from build123d import *

# Parameters (mm, degrees)
SKETCH1_W           = 275
SKETCH1_H           = 200
BOSS_EXTRUDE1_DEPTH = 1.5
SKETCH3_W           = 275
SKETCH3_H           = 200
SKETCH3_W_2         = 272
SKETCH3_H_2         = 197
BOSS_EXTRUDE2_DEPTH = 55
SKETCH4_R           = 1.5
SKETCH4_R_2         = 6.1
MOUNT_HOLE_DEPTH    = 250


with BuildPart() as part:
    # Sketch1 → Boss-Extrude1 (new body)
    with BuildSketch(Plane(origin=(0, 0, 0), x_dir=(1, 0, 0), z_dir=(0, 1, 0))):
        Rectangle(SKETCH1_W, SKETCH1_H)
    extrude(amount=BOSS_EXTRUDE1_DEPTH)

    # Sketch3 → Boss-Extrude2 (add)
    with BuildSketch(Plane(origin=(0, 1.5, 0), x_dir=(1, 0, 0), z_dir=(0, 1, 0))):
        Rectangle(SKETCH3_W, SKETCH3_H)
        Rectangle(SKETCH3_W_2, SKETCH3_H_2, mode=Mode.SUBTRACT)
    extrude(amount=BOSS_EXTRUDE2_DEPTH)

    # Sketch4 → MOUNT HOLE (cut)
    with BuildSketch(Plane(origin=(0, 0, -100), x_dir=(-1, 0, 0), z_dir=(0, 0, -1))):
        with Locations((-47, 28.25)):
            Circle(SKETCH4_R)
        with Locations((-54.75, 14.826606241)):
            Circle(SKETCH4_R)
        with Locations((-70.25, 14.826606241)):
            Circle(SKETCH4_R)
        with Locations((-78, 28.25)):
            Circle(SKETCH4_R)
        with Locations((-70.25, 41.673393759)):
            Circle(SKETCH4_R)
        with Locations((-54.75, 41.673393759)):
            Circle(SKETCH4_R)
        with Locations((78, 28.25)):
            Circle(SKETCH4_R)
        with Locations((70.25, 14.826606241)):
            Circle(SKETCH4_R)
        with Locations((54.75, 14.826606241)):
            Circle(SKETCH4_R)
        with Locations((47, 28.25)):
            Circle(SKETCH4_R)
        with Locations((54.75, 41.673393759)):
            Circle(SKETCH4_R)
        with Locations((70.25, 41.673393759)):
            Circle(SKETCH4_R)
        with Locations((-62.5, 21.5)):
            Circle(SKETCH4_R_2)
        with Locations((62.5, 21.5)):
            Circle(SKETCH4_R_2)
    extrude(amount=-MOUNT_HOLE_DEPTH, mode=Mode.SUBTRACT)


solid = part.part
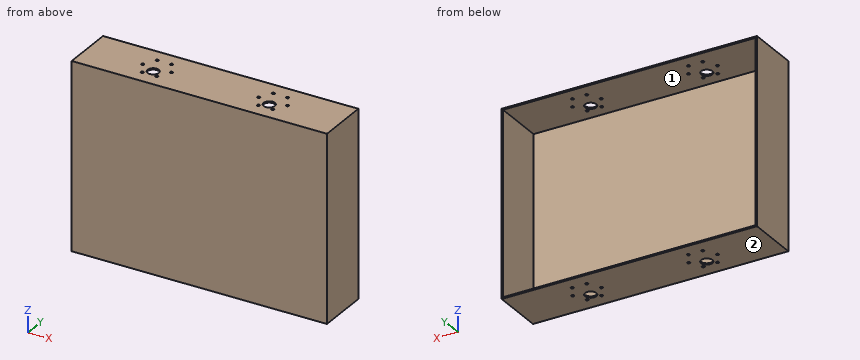
Read the model definition and answer for the solid it produces. Units are mm, in the model's axes. Face numbers are marked on the shaded views. A direction names the side the tool comes from. Give positions to 0.01 mm unless a question says otherwise; leave off trailing zeros. Write each loop counter-clockwise with the first axis right and the second up, starting at its lowest first coordinate (ties: lowest second). Pieces come first, ordered by that corner, then holes. Notation, with made-up numbers: (-27, -26) - (26, -26) arc R15 ccw to (26, 1) - close; hole circle Ø4 at (71.5, -8). An arc over 180 degrees is marked (long way). Answer in a Markdown table with one row per item. Add a question column.
Item 1: Section A-A, the plane z = -10 is taken. Write down the section's boundary in (x, y).
Item 2: Section C-C, the plane y = 9.5 is taken. Write down the section's boundary in (x, z).
Item 3: Find the intervals of material crossed by L1, parallel to X at y = 21, z = 99; L2, parallel to Y at x = 54.75, z = -99.3; L3, parallel to Z at x = -2.5, y = 15, in increasing order.
Item 4: A flat-ended cylindrical pin translates along its axis: P1, Ø3, axis at x = 29, z = -29, coming from the +Y side. Find the tip coordinate at first contact, or state that the pin passes through.
Item 5: A tool of negligible diameter and unlimited length cuts with its end or side. For the marked faces 1 and 2, from which of +Z, -Z, +X, -X, +Y, -Y can it reach the whole face along a straight path? Write none if from no direction.
Item 6: Section B-B, the plane x = 7 is taken. Write down the section's boundary in (y, z).
Recorded:
| question | item | result |
|---|---|---|
| 1 | outline | (-137.5, 0) - (137.5, 0) - (137.5, 56.5) - (136, 56.5) - (136, 1.5) - (-136, 1.5) - (-136, 56.5) - (-137.5, 56.5) - close |
| 2 | outline | (-137.5, -100) - (137.5, -100) - (137.5, 100) - (-137.5, 100) - close; hole (-136, -98.5) - (136, -98.5) - (136, 98.5) - (-136, 98.5) - close |
| 3 | L1 | x = -137.5 to -68.58, -56.42 to 56.42, 68.58 to 137.5 |
| 3 | L2 | y = 0 to 13.33, 16.33 to 40.17, 43.17 to 56.5 |
| 3 | L3 | z = -100 to -98.5, 98.5 to 100 |
| 4 | P1 | stops at y = 1.5 |
| 5 | face 1 | +Y |
| 5 | face 2 | -Z, +X, -X, +Y, -Y |
| 6 | outline | (0, -100) - (56.5, -100) - (56.5, -98.5) - (1.5, -98.5) - (1.5, 98.5) - (56.5, 98.5) - (56.5, 100) - (0, 100) - close |
